from build123d import *

# Parameters (mm, degrees)
F1_DEPTH = 10
F2_T     = -2
F3_W     = 10
F3_H     = 90
F4_DEPTH = 2
F5_R     = 2


with BuildPart() as f1:
    # F0 (on Right) → F1 (new body, symmetric)
    with BuildSketch(Plane.YZ):
        Polygon((-0.131682, 59.474063), (-10.131682, 59.474063), (-10.131682, -0.525937), (-16.131682, -0.525937), (-16.131682, -40.525937), (-0.131682, -40.525937), align=None)
    extrude(amount=F1_DEPTH, both=True)

    # F2
    f2_openings = [f1.faces().sort_by_distance(p)[0] for p in [
        (0, -13.131682, -0.525937),
        (0, -10.131682, 29.474063),
        (0, -5.131682, 59.474063),
        (10, -6.680069, 3.667611),
        (-10, -6.680069, 3.667611),
    ]]
    offset(amount=F2_T, openings=f2_openings)

    # F3 (on face) → F4 (cut)
    with BuildSketch(Plane(origin=(0, -0.131682, 0), x_dir=(-1, 0, 0), z_dir=(0, 1, 0))):
        with Locations((0, 9.474063)):
            Rectangle(F3_W, F3_H)
    extrude(amount=-F4_DEPTH, mode=Mode.SUBTRACT)

    # F5
    f5_edges = [f1.edges().sort_by_distance(p)[0] for p in [
        (10, -1.131682, 59.474063),
        (-10, -1.131682, 59.474063),
        (-5, -1.131682, 54.474063),
        (5, -1.131682, 54.474063),
        (0, -0.131682, -40.525937),
        (0, -16.131682, -40.525937),
        (-5, -1.131682, -35.525937),
        (5, -1.131682, -35.525937),
    ]]
    fillet(f5_edges, radius=F5_R)


solid = f1.part
Source: CAD feature listing. Evaluate the final solid. Frame: model axes, mm. A direction names the side the tool comes from. Round coordinates to 2 decimals unless told otherwise and drop trailing zeros. Order: outer loops, then holes, each group sorted by start corner. A loop starts at its lowest first (then second) coordinate and runs counter-clockwise, first axis right, second up. Notation, with made-up numbers: (-1, -30.5) - (55, -30.5) arc R27 ccw to (55, -13.5) - close; hole circle Ø4 at (71, 81). An arc over 180 degrees is marked (long way). Use a Markdown table: item, result. Add a question column.
1. Line query: probe 1 along Y at (x, z) = (8, -17.5); probe 2 along X at (y, z) = (-1.5, -32.5); probe 3 along Y at (x, z) = (5.5, 43.5). Output: solid intervals per line, ascending.
2. Section query D-D (y = -3.5). Return the cut outline in (x, z), then the cut area to 3 significant figures.
3. Section query B-B (x = 0.5). Return the cut outline in (y, z).
4. Section query C-C (z = -29). Return the cut outline in (x, y).
5. Mould query, pull axis Z, two halves, no side actions, for faces 1 (the flat face through (10, -1.7, 1.4)), 2 (the cylindrical face through (-4.399, -1.146, -34.956)), 3 (the cylindrical face through (9.4, -1.1, 58.9)). Classes: +Z half, -Z half, draft (parallel to the pull), parting line (faces both ways), or undercut.
6. Section query A-A (z = 43). Return the cut outline in (x, y), then the cut area to 3 significant figures.
7. Set-up query: faces 4 (the flat face through (7, -2.132, 10)), 5 (the flat face through (-5, -1, 9)), 6 (the flat face through (0, -15, -0.526)), 7 (the cylindrical face through (4.4, -1.1, 53.9)). Return all of +Z, -Z, +X, -X, +Y, -Y with unobstructed straight access to the full face (end or side cutting, diameter ignored); none if empty.
8. First-contact query: pin 1 (1 mm diameter, centred on x = 0, y = -1, fed in from -Z); pin 2 (3 mm diameter, centred on x = -5, z = 47.5, fed in from -Y); pin 3 (6 mm diameter, centred on x = 2.5, y = -8.5, fed in from +Z). Flat tips, straight axial feed; report the tip coordinate or a pass-through.
Derived:
| question | item | result |
|---|---|---|
| 1 | probe 1 | -16.13 to -14.13, -2.13 to -0.13 |
| 1 | probe 2 | -10 to -5, 5 to 10 |
| 1 | probe 3 | -2.13 to -0.13 |
| 2 | outline | (-10, -40.53) - (10, -40.53) - (10, -38.53) - (-10, -38.53) - close |
| 2 | area | 40.0 mm2 |
| 3 | outline | (-16.13, -38.53) arc R2 ccw to (-14.13, -40.53) - (-2.13, -40.53) arc R2 ccw to (-0.13, -38.53) - (-0.13, -35.53) - (-2.13, -35.53) - (-2.13, -38.53) - (-14.13, -38.53) - (-14.13, -0.53) - (-16.13, -0.53) - close; (-2.13, 54.47) - (-0.13, 54.47) - (-0.13, 59.47) - (-2.13, 59.47) - close |
| 4 | outline | (-10, -16.13) - (10, -16.13) - (10, -14.13) - (-10, -14.13) - close; (-10, -2.13) - (-5, -2.13) - (-5, -0.13) - (-10, -0.13) - close; (5, -2.13) - (10, -2.13) - (10, -0.13) - (5, -0.13) - close |
| 5 | face 1 | draft |
| 5 | face 2 | undercut |
| 5 | face 3 | +Z half |
| 6 | outline | (-10, -2.13) - (-5, -2.13) - (-5, -0.13) - (-10, -0.13) - close; (5, -2.13) - (10, -2.13) - (10, -0.13) - (5, -0.13) - close |
| 6 | area | 20.0 mm2 |
| 7 | face 4 | +Z, +X, -X |
| 7 | face 5 | +Y |
| 7 | face 6 | +Z, +X, -X, -Y |
| 7 | face 7 | +Y, -Y |
| 8 | pin 1 | z = -40.42 |
| 8 | pin 2 | y = -2.13 |
| 8 | pin 3 | z = -38.53 |
